Geometry check sheet. Reference: the model listing, model coordinates, mm. A direction names the side the tool comes from. Give positions to 0.01 mm unless a question says otherwise; leave off trailing zeros. Write each loop counter-clockwise with the first axis right and the second up, starting at its lowest first coordinate (ties: lowest second). Pieces come first, ordered by that corner, then holes.
(1) Cross-section at C-C (x = -9). Record the boundary of the cut face in (y, z).
(2) Tool access check on faces 5 (the flat face through (7.09, 15.24, 42.21)), 6 (the cylindrical face through (-16.505, 16.392, 25.044)). Record the directions out of +Z, -Z, +X, -X, +Y, -Y that give a thin tool (end or side, any length) a straight path to the whole face; none if there is none.
(3) Thickness scan on line 1 along X through (y, z) = (-2.5, 3); line 2 along X through (y, z) = (-8, 41); line 3 along Y through (x, z) = (40, 40). Record the ranges inside material, lowest first.
(4) Mould release check, pull along X, two halves, no side actions. Record for faces 1 (the flat face through (1, 13, 50.8)), 2 (the cylindrical face through (-4.087, 16.549, 26.716)), 3 (the cylindrical face through (-0.27, 11.49, 25.04)), 4 (the flat face through (-72.172, -15.601, 25.044)): +X half, -X half, draft (parallel to the pull), parting line (faces both ways), or undercut.
(5) Cross-section at A-A (y = 8). Record the boundary of the cut face in (x, z), and give its area (3 significant figures).
(6) Depth check by flat-ended pin: P1, Ø6.5, axis at x = -3.26, z = 34.1, coming from the +Y side; P2, Ø1.5, axis at x = -37, z = 5.5, coming from the -Y side; P3, Ø6, axis at y = -7, z = 45.5, coming from the +X side. Enter the tip coordinate at first touch or a pass-through.
(7) Cross-section at B-B (z = 17). Record the boundary of the cut face in (x, y), and give its area (3 significant figures).
(8) Cross-section at D-D (y = -10.5). Record the boundary of the cut face in (x, z).
```python
from build123d import *

# Parameters (mm, degrees)
F1_DEPTH = 50.8
F3_R     = 18.840959
F3_R_2   = 15.518861
F4_DEPTH = 5.08


with BuildPart() as f1:
    # F0 (on Top) → F1 (new body)
    with BuildSketch(Plane.XY):
        with BuildLine():
            Line((71.684018, -17.545537), (76.151238, -13.032617))
            ThreePointArc((76.151238, -13.032617), (0.810028, 17.846849), (-74.385113, -13.386627))
            Line((-74.385113, -13.386627), (-69.896718, -17.878487))
            ThreePointArc((-69.896718, -17.878487), (0.824961, 11.496866), (71.684018, -17.545537))
        make_face()
    extrude(amount=F1_DEPTH)

    # F3 (on offset) → F4 (cut)
    with BuildSketch(Plane.XZ.offset(-20.32)):
        with Locations((4.391287, 26.769793)):
            Circle(F3_R)
        with Locations((4.391287, 26.769793)):
            Circle(F3_R_2, mode=Mode.SUBTRACT)
        with BuildLine():
            ThreePointArc((-4.417794, 21.524068), (-4.064254, 26.78749), (-1.260601, 31.256061))
            ThreePointArc((-1.260601, 31.256061), (-1.442666, 37.063663), (-6.704263, 34.598508))
            ThreePointArc((-6.704263, 34.598508), (-6.685209, 27.864691), (-4.417794, 21.524068))
        make_face()
        with BuildLine():
            ThreePointArc((3.559272, 37.963443), (7.940759, 35.025558), (10.408828, 30.363238))
            ThreePointArc((10.408828, 30.363238), (15.529392, 27.617109), (16.025304, 33.406364))
            ThreePointArc((16.025304, 33.406364), (10.18412, 36.756771), (3.559272, 37.963443))
        make_face()
        with BuildLine():
            ThreePointArc((13.262496, 23.655856), (8.527469, 21.33032), (3.255747, 21.524069))
            ThreePointArc((3.255747, 21.524069), (-1.682752, 18.462594), (3.082934, 15.138495))
            ThreePointArc((3.082934, 15.138495), (8.905063, 18.521906), (13.262496, 23.655856))
        make_face()
    extrude(amount=F4_DEPTH, mode=Mode.SUBTRACT)


solid = f1.part
```
Reply:
1. outline: (10.99, 0) - (17.37, 0) - (17.37, 13.52) - (15.24, 13.52) - (15.24, 18.93) - (17.37, 18.93) - (17.37, 34.61) - (15.24, 34.61) - (15.24, 40.02) - (17.37, 40.02) - (17.37, 50.8) - (10.99, 50.8) - close
2. face 5: +Y
2. face 6: +Z, -Z, +Y
3. line 1: x = -61.63 to -50.07, 52.19 to 63.75
3. line 2: x = -68.58 to -58.39, 60.51 to 70.7
3. line 3: y = 3.64 to 10.49
4. face 1: draft
4. face 2: undercut
4. face 3: undercut
4. face 4: -X half
5. outline: (-43.72, 0) - (-25.21, 0) - (-25.21, 50.8) - (-43.72, 50.8) - close; (27.33, 0) - (45.84, 0) - (45.84, 50.8) - (27.33, 50.8) - close
5. area: 1,880 mm2
6. P1: stops at y = 15.24
6. P2: stops at y = 3.69
6. P3: stops at x = 72.96
7. outline: (-74.39, -13.39) - (-69.9, -17.88) arc R100.39 cw to (71.68, -17.55) - (76.15, -13.03) arc R106.74 ccw to (20.5, 16.06) - (20.5, 15.24) - (16.45, 15.24) - (16.45, 16.73) arc R106.74 ccw to (6.83, 17.69) - (6.83, 15.24) - (-1.4, 15.24) - (-1.4, 17.82) arc R106.74 ccw to (-7.67, 17.49) - (-7.67, 15.24) - (-11.72, 15.24) - (-11.72, 17.08) arc R106.74 ccw to start
7. area: 995 mm2
8. outline: (-71.38, 0) - (-61.65, 0) - (-61.65, 50.8) - (-71.38, 50.8) - close; (63.77, 0) - (73.5, 0) - (73.5, 50.8) - (63.77, 50.8) - close
